Design review of the part shown in the three views and the two pictorial views. Dimensions are in mm from the part's minimum x, y and z. Coordinates: 2 decimals unless noted, no trailing zeros. Order: outer loops, then holes, each group sorted by start corner. A loop starts at its lowest first (then second) coordinate and runs counter-clockwise, first axis right, second up. Notation, with made-up numbers: (13, 34.5) - (18, 34.5) arc R34 ccw to (18, 70.5) - close; hole circle Ø11 at (-22, 35). An arc over 180 degrees is marked (long way). One line per item, written item: value. Start each with the question number.
(1) Mouldability with a two-part tool opening along X and no side actions: class the marked faces 1, 2, 3 and 4 as released by +X, released by -X, zero draft, split by the parting line, or undercut.
(2) To check wall thickness, follow line 1 along Y through (x, z) = (19.05, 2.7); line 2 along Y through (x, z) = (6, 2.5); line 3 along X through (y, z) = (14, 3.95) (1 decimal). State the ranges of each line that lie inside material, in increasing order.
(3) Consider section D-D on z = 4.8. Count the separate pieces of the cut face and the enclosed holes in it, then the cut area to 3 significant figures.
(4) Consider section C-C on x = 12. Write out the cut boundary in (y, z), then the cut area to 3 significant figures.
(5) Consider section A-A on y = 19.05. Write out the cut boundary in (x, z), then the cut area to 3 significant figures.
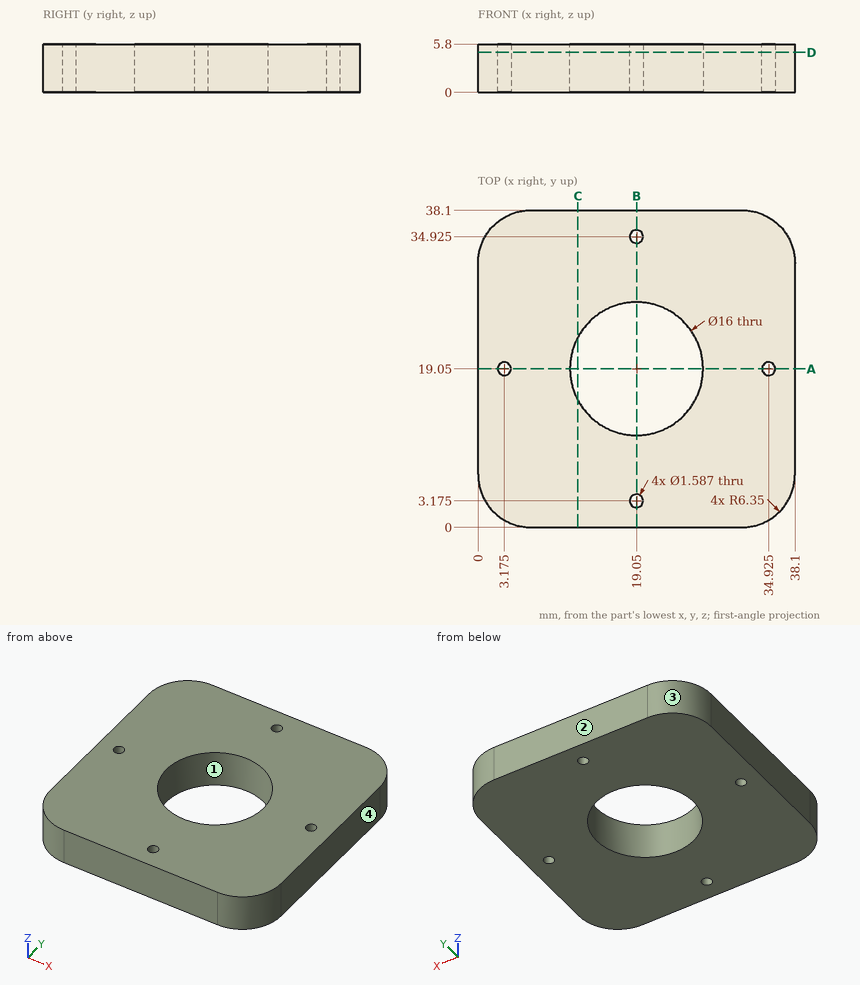
Geometry check:
1. face 1: undercut
1. face 2: zero draft
1. face 3: released by -X
1. face 4: released by +X
2. line 1: y = 0 to 2.38, 3.97 to 11.05, 27.05 to 34.13, 35.72 to 38.1
2. line 2: y = 0.01 to 38.09
2. line 3: x = 0 to 12.8, 25.3 to 38.1
3. separate pieces: 1
3. enclosed holes: 5
3. area: 1,210 mm^2
4. outline: (0, 0) - (15.27, 0) - (15.27, 5.8) - (0, 5.8) - close; (22.83, 0) - (38.1, 0) - (38.1, 5.8) - (22.83, 5.8) - close
4. area: 177 mm^2
5. outline: (0, 0) - (2.38, 0) - (2.38, 5.8) - (0, 5.8) - close; (3.97, 0) - (11.05, 0) - (11.05, 5.8) - (3.97, 5.8) - close; (27.05, 0) - (34.13, 0) - (34.13, 5.8) - (27.05, 5.8) - close; (35.72, 0) - (38.1, 0) - (38.1, 5.8) - (35.72, 5.8) - close
5. area: 110 mm^2
